from build123d import *

# Parameters (mm, degrees)
SKETCH3_R           = 7.7216
SKETCH3_R_2         = 6.13382221
BOSS_EXTRUDE1_DEPTH = 7.112
CHAMFER1_SIZE       = 1.27


with BuildPart() as part:
    # Sketch1 → Revolve1 (revolve)
    with BuildSketch(Plane(origin=(0, 0, 0), x_dir=(0, 0, -1), z_dir=(1, 0, 0))):
        Polygon((0, 152.4), (0, 0), (-10.57275, 0), (-7.7216, 152.4), align=None)
    revolve(axis=Axis((0, 152.4, 0), (0, -1, 0)))

    # Sketch2 → Cut-Revolve4 (revolve, cut)
    with BuildSketch(Plane(origin=(0, 0, 0), x_dir=(0, 0, -1), z_dir=(1, 0, 0))):
        Polygon((0, 152.4), (0, 0), (-8.98497221, 0), (-6.13382221, 152.4), align=None)
    revolve(axis=Axis((0, 287.681750321, 0), (0, -1, 0)), mode=Mode.SUBTRACT)

    # Sketch3 → Boss-Extrude1 (add)
    with BuildSketch(Plane(origin=(0, 152.4, 0), x_dir=(1, 0, 0), z_dir=(0, 1, 0))):
        with Locations(Location((0, 0, 0), (0, 0, 270))):
            Circle(SKETCH3_R)
        with Locations(Location((0, 0, 0), (0, 0, 270))):
            Circle(SKETCH3_R_2, mode=Mode.SUBTRACT)
    extrude(amount=BOSS_EXTRUDE1_DEPTH)

    # Chamfer1
    chamfer1_edges = [part.edges().sort_by_distance(p)[0] for p in [
        (0, 159.512, -6.13382221),
    ]]
    chamfer(chamfer1_edges, length=CHAMFER1_SIZE)


solid = part.part
Model file for the job. Use its own axes, mm. A direction names the side the tool comes from. Give positions to 0.01 mm unless a question says otherwise; leave off trailing zeros. Loops run counter-clockwise (first coordinate to the right, second up) from the corner with the lowest first, then second, coordinate; pieces in that order, holes last.
1) Tool access for faces 4 (the conical face through (-7.7, 77.3, 4.9)), 5 (the conical face through (7.36, 77.27, -1.63)): list every direction of +Z, -Z, +X, -X, +Y, -Y with a clear straight run to the whole face (end or side of a thin tool).
2) Flat gauge pins, fed straight in: pin 1 Ø2 at (x, y) = (4, 113.5) entering from -Z; pin 2 Ø6 at (x, y) = (3, 40.5) entering from +Z; pin 3 Ø5 at (y, z) = (86, 5.5) entering from -X. Where does each tip first touch, or does it go through?
3) Pull direction Z, two halves, no side cores. Call faces 1 (the flat face through (8, 0, 5)), 2 (the cylindrical face through (7.656, 155.906, -1.005)), 3 (the cylindrical face through (-3.73, 155.28, -4.87)): +Z half, -Z half, draft (parallel to the pull), parting line (faces both ways), or undercut.
4) Saw through at B-B (y = 140.5). Write the cut outline in (x, z).
5) Saw through at A-A (y = 19.5). Write the cut outline in (x, z), plus the area to 3 significant figures.
6) Wall check: line 1 (X direction, y = 157, z = 0); line 2 (Z direction, x = -4.5, y = 80). Give the ranges that are in metal, low to high.
Answer block:
1. face 4: +Y
1. face 5: -Y
2. pin 1: stops at z = -7.9
2. pin 2: stops at z = 9.84
2. pin 3: stops at x = -8.45
3. face 1: draft
3. face 2: parting line
3. face 3: undercut
4. outline: circle Ø15.89 at (0, 0); hole circle Ø12.71 at (0, 0)
5. outline: circle Ø20.42 at (0, 0); hole circle Ø17.24 at (0, 0)
5. area: 93.9 mm2
6. line 1: x = -7.72 to -6.13, 6.13 to 7.72
6. line 2: z = -7.88 to -5.99, 5.99 to 7.88
